Work out the finished part from the listing and answer in its coordinate system (mm). A direction names the side the tool comes from. Give positions to 0.01 mm unless a question says otherwise; leave off trailing zeros. Write each loop counter-clockwise with the first axis right and the second up, starting at its lowest first coordinate (ties: lowest second). Pieces come first, ordered by that corner, then holes.
1) Given pin 1 Ø2 at (y, z) = (0.5, 1) entering from +X (3 decimals); pin 2 Ø1.5 at (x, z) = (0, 1.5) entering from -Y; pin 3 Ø2.5 at (x, z) = (8, -0.5) entering from -Y, each flat-ended and moving along its own axis, determine where each tip first touches the part or whether it passes through.
2) Find section D-D (y = 0.8). Determine the outline of the cut face in (x, z) (3 decimals), plus the area to 3 significant figures.
3) Straight lines are drawn through the part: probe 1 along Y at (x, z) = (-1.5, 1.75); probe 2 along X at (y, z) = (2.6, 0) (3 decimals); probe 3 along X at (y, z) = (2.95, 1). For each, find the intervals that lie inside material, in ascending order.
4) A tool of negligible diameter and unlimited length cuts with its end or side. For faces 5 (the face through (-1, 3, 1)), 6 (the face through (6.786, 3.316, -0.065)), 7 (the face through (-3.307, 1.972, 0.434)), from which of +Z, -Z, +X, -X, +Y, -Y can it reach the whole face along a straight path? Write none if from no direction.
5) Find section A-A (x = 0). Determine the outline of the cut face in (y, z) (3 decimals), plus the area to 4 significant figures.
6) Determine the mould class of faces 1 (the face through (12.786, 3.316, -0.065)), 2 (the face through (10.786, 3.316, -0.065)), 3 (the face through (8.331, 3.316, 2.232)), 4 (the face through (16.168, 3.316, -0.04)) for opening direction Z: pulls with the +Z half, pulls with the -Z half, needs draft (parallel to the pull), parting line crosses it, or undercut.
7) Find section B-B (y = 3.25). Count the separate pieces of the cut face and the enclosed holes in it, plus the area to 3 significant figures.
```python
from build123d import *

# Parameters (mm, degrees)
BOSS_EXTRUDE1_START = -1.35
SKETCH3_R           = 0.5
BOSS_EXTRUDE1_DEPTH = 1.35


with BuildPart() as part:
    # Sketch2 → Revolve1 (revolve)
    with BuildSketch(Plane.XY, mode=Mode.PRIVATE) as revolve1_sk:
        Polygon((2.45, 0), (2.45, 2.25), (1.2, 2.25), (1.2, 3), (2.45, 3), (2.45, 4), (3.335, 4), (3.335, 0), align=None)
    revolve(revolve1_sk.sketch.rotate(Axis((0, 0, 0), (0, 1, 0)), 90), axis=Axis((0, 0, 0), (0, 1, 0)))

    # Sketch3 → Boss-Extrude1 (add)
    with BuildSketch(Plane(origin=(0, 4, 0), x_dir=(1, 0, 0), z_dir=(0, 1, 0)).offset(BOSS_EXTRUDE1_START)):
        with BuildLine():
            Line((2.088594025, 2.6), (14.400412206, 1.875))
            ThreePointArc((14.400412206, 1.875), (16.168248081, 0), (14.400412206, -1.875))
            Line((14.400412206, -1.875), (2.088594025, -2.6))
            ThreePointArc((2.088594025, -2.6), (3.335, 0), (2.088594025, 2.6))
        make_face()
        with Locations(Location((14.29, 0, 0), (0, 0, 270))):
            Circle(SKETCH3_R, mode=Mode.SUBTRACT)
        with Locations(Location((12.29, 0, 0), (0, 0, 270))):
            Circle(SKETCH3_R, mode=Mode.SUBTRACT)
        with Locations(Location((10.29, 0, 0), (0, 0, 270))):
            Circle(SKETCH3_R, mode=Mode.SUBTRACT)
        with Locations(Location((8.29, 0, 0), (0, 0, 270))):
            Circle(SKETCH3_R, mode=Mode.SUBTRACT)
        with Locations(Location((6.29, 0, 0), (0, 0, 270))):
            Circle(SKETCH3_R, mode=Mode.SUBTRACT)
        with Locations(Location((4.29, 0, 0), (0, 0, 270))):
            Circle(SKETCH3_R, mode=Mode.SUBTRACT)
    extrude(amount=BOSS_EXTRUDE1_DEPTH)


solid = part.part
```
Results:
1. pin 1: stops at x = 3.335
1. pin 2: stops at y = 2.25
1. pin 3: stops at y = 2.65
2. outline: circle Ø6.67 at (0, 0); hole circle Ø4.9 at (0, 0)
2. area: 16.1 mm2
3. probe 1: y = 2.25 to 3
3. probe 2: x = -3.335 to -1.2, 1.2 to 3.335
3. probe 3: x = -3.18 to -0.66, 0.66 to 15.88
4. face 5: +Y
4. face 6: +Y, -Y
4. face 7: -Y
5. outline: (0, -3.335) - (4, -3.335) - (4, -2.45) - (3, -2.45) - (3, -1.2) - (2.25, -1.2) - (2.25, -2.45) - (0, -2.45) - close; (0, 2.45) - (2.25, 2.45) - (2.25, 1.2) - (3, 1.2) - (3, 2.45) - (4, 2.45) - (4, 3.335) - (0, 3.335) - close
5. area: 8.955 mm2
6. face 1: undercut
6. face 2: undercut
6. face 3: pulls with the +Z half
6. face 4: parting line crosses it
7. separate pieces: 1
7. enclosed holes: 7
7. area: 67.1 mm2
